Source: CAD feature listing. Evaluate the final solid. Frame: model axes, mm. A direction names the side the tool comes from. Give positions to 0.01 mm unless a question says otherwise; leave off trailing zeros. Order: outer loops, then holes, each group sorted by start corner. A loop starts at its lowest first (then second) coordinate and runs counter-clockwise, first axis right, second up. Notation, with made-up numbers: (39, 51.5) - (73, 51.5) arc R21 cw to (73, 82.5) - close; hole circle Ø1 at (59.5, 26). An arc over 180 degrees is marked (long way). Write each question's results on one line, items separated by ' | '. Start each with the question number.
Item 1: Section C-C on z = 5. Output: boundary loops of the cut face in (x, y), and give its area (3 significant figures).
Item 2: Section A-A on x = 49. Output: boundary loops of the cut face in (y, z).
Item 3: Mould query, pull axis X, two halves, no side actions, for faces 4 (the flat face through (0, 5, 20)), 5 (the flat face through (95, 0, 20)), 6 (the flat face through (50, 5, 30)), 7 (the flat face through (26, 5, 20)). Classes: released by +X, released by -X, zero draft, split by the parting line, or undercut.
Item 4: Section B-B on x = 95. Output: boundary loops of the cut face in (y, z).
Item 5: Line query: line 1 along Z through (x, y) = (95, 6); line 2 along X through (y, z) = (3.5, 5); line 3 along Z through (x, y) = (47, 5.5). Output: solid intervals per line, ascending.
Item 6: Contact query for a flat-ended pin moving along its axis: pin 1 Ø3 at (x, z) = (12, 25) entering from -Y. Output: stop coordinate, or through.
Item 7: Section D-D on y = 5.5. Output: boundary loops of the cut face in (x, z), and give its area (3 significant figures).
Item 8: Set-up query: faces 1 (the flat face through (10, 1, 20)), 2 (the flat face through (49, 5, 0)), 3 (the flat face through (50, 5, 10)). Return all of +Z, -Z, +X, -X, +Y, -Y with unobstructed straight access to the full face (end or side cutting, diameter ignored); none if empty.
```python
from build123d import *

# Parameters (mm, degrees)
BOSS_EXTRU_1_DEPTH      = 40
ENL_V_MAT_EXTRU_1_REACH = 110.167
ESQUISSE2_W             = 48
ESQUISSE2_H             = 20
ENL_V_MAT_EXTRU_2_REACH = 110.167
ESQUISSE3_R             = 1.25


with BuildPart() as part:
    # Esquisse1 → Boss.-Extru.1 (new body)
    with BuildSketch(Plane.XY):
        Polygon((0, 0), (10, 0), (10, 3), (16, 3), (16, 0), (84, 0), (84, 3), (90, 3), (90, 0), (100, 0), (100, 10), (0, 10), align=None)
    extrude(amount=BOSS_EXTRU_1_DEPTH)

    # Esquisse2 → Enlèv. mat.-Extru.1 (cut, up to next)
    with BuildSketch(Plane(origin=(0, 10, 0), x_dir=(1, 0, 0), z_dir=(0, 1, 0)), mode=Mode.PRIVATE) as enl_v_mat_extru_1_sk1:
        with Locations((50, -20)):
            Rectangle(ESQUISSE2_W, ESQUISSE2_H)
    enl_v_mat_extru_1_tool1 = extrude(enl_v_mat_extru_1_sk1.sketch, amount=-ENL_V_MAT_EXTRU_1_REACH, mode=Mode.PRIVATE) & part.part
    add(enl_v_mat_extru_1_tool1.solids().sort_by_distance((50, 10, 20))[0], mode=Mode.SUBTRACT)

    # Esquisse3 → Enlèv. mat.-Extru.2 (cut, up to next)
    with BuildSketch(Plane.XZ, mode=Mode.PRIVATE) as enl_v_mat_extru_2_sk1:
        with Locations(Location((5, 35, 0), (0, 0, 270))):
            Circle(ESQUISSE3_R)
    enl_v_mat_extru_2_tool1 = extrude(enl_v_mat_extru_2_sk1.sketch, amount=-ENL_V_MAT_EXTRU_2_REACH, mode=Mode.PRIVATE) & part.part
    # Esquisse3 → Enlèv. mat.-Extru.2 (cut, up to next)
    with BuildSketch(Plane.XZ, mode=Mode.PRIVATE) as enl_v_mat_extru_2_sk2:
        with Locations(Location((5, 5, 0), (0, 0, 270))):
            Circle(ESQUISSE3_R)
    enl_v_mat_extru_2_tool2 = extrude(enl_v_mat_extru_2_sk2.sketch, amount=-ENL_V_MAT_EXTRU_2_REACH, mode=Mode.PRIVATE) & part.part
    # Esquisse3 → Enlèv. mat.-Extru.2 (cut, up to next)
    with BuildSketch(Plane.XZ, mode=Mode.PRIVATE) as enl_v_mat_extru_2_sk3:
        with Locations(Location((95, 35, 0), (0, 0, 270))):
            Circle(ESQUISSE3_R)
    enl_v_mat_extru_2_tool3 = extrude(enl_v_mat_extru_2_sk3.sketch, amount=-ENL_V_MAT_EXTRU_2_REACH, mode=Mode.PRIVATE) & part.part
    # Esquisse3 → Enlèv. mat.-Extru.2 (cut, up to next)
    with BuildSketch(Plane.XZ, mode=Mode.PRIVATE) as enl_v_mat_extru_2_sk4:
        with Locations(Location((95, 5, 0), (0, 0, 270))):
            Circle(ESQUISSE3_R)
    enl_v_mat_extru_2_tool4 = extrude(enl_v_mat_extru_2_sk4.sketch, amount=-ENL_V_MAT_EXTRU_2_REACH, mode=Mode.PRIVATE) & part.part
    add(enl_v_mat_extru_2_tool1.solids().sort_by_distance((5, 0, 35))[0], mode=Mode.SUBTRACT)
    add(enl_v_mat_extru_2_tool2.solids().sort_by_distance((5, 0, 5))[0], mode=Mode.SUBTRACT)
    add(enl_v_mat_extru_2_tool3.solids().sort_by_distance((95, 0, 35))[0], mode=Mode.SUBTRACT)
    add(enl_v_mat_extru_2_tool4.solids().sort_by_distance((95, 0, 5))[0], mode=Mode.SUBTRACT)


solid = part.part
```
Evaluation:
1) outline: (0, 0) - (3.75, 0) - (3.75, 10) - (0, 10) - close; (6.25, 0) - (10, 0) - (10, 3) - (16, 3) - (16, 0) - (84, 0) - (84, 3) - (90, 3) - (90, 0) - (93.75, 0) - (93.75, 10) - (6.25, 10) - close; (96.25, 0) - (100, 0) - (100, 10) - (96.25, 10) - close | area: 914 mm^2
2) outline: (0, 0) - (10, 0) - (10, 10) - (0, 10) - close; (0, 30) - (10, 30) - (10, 40) - (0, 40) - close
3) face 4: released by -X | face 5: zero draft | face 6: undercut | face 7: undercut
4) outline: (0, 0) - (10, 0) - (10, 3.75) - (0, 3.75) - close; (0, 6.25) - (10, 6.25) - (10, 33.75) - (0, 33.75) - close; (0, 36.25) - (10, 36.25) - (10, 40) - (0, 40) - close
5) line 1: z = 0 to 3.75, 6.25 to 33.75, 36.25 to 40 | line 2: x = 0 to 3.75, 6.25 to 93.75, 96.25 to 100 | line 3: z = 0 to 10, 30 to 40
6) pin 1: stops at y = 3
7) outline: (0, 0) - (100, 0) - (100, 40) - (0, 40) - close; hole circle Ø2.5 at (5, 5); hole circle Ø2.5 at (5, 35); hole (26, 10) - (74, 10) - (74, 30) - (26, 30) - close; hole circle Ø2.5 at (95, 5); hole circle Ø2.5 at (95, 35) | area: 3,020 mm^2
8) face 1: +Z, -Z, -Y | face 2: -Z, +X, -X, +Y, -Y | face 3: +Y, -Y
